Geometry: final body of the model. Coordinates: model frame, mm. Face numbers are marked on the shaded views. A direction names the side the tool comes from. Give positions to 0.01 mm unless a question says otherwise; leave off trailing zeros. Write each loop counter-clockwise with the first axis right and the second up, starting at its lowest first coordinate (ties: lowest second). Pieces come first, ordered by that corner, then holes. Notation, with made-up numbers: M 38,24 L 84,24 A19 ccw 84,54 Z; hole C 81,33 d2. An arc over 180 degrees is marked long. Use one line per item in the form item = value. Start each with the question number.
Item 1: Access query for the marked faces 5, 6 and 7. Directions: +Z, -Z, +X, -X, +Y, -Y. A direction counts if a zero-diameter tool reaches every point of the face in a straight line with its end or side. Return the directions, or none.
Item 2: Material intervals for line 1 along Z through (x, y) = (110, 6.5); line 2 along X through (y, z) = (11.5, -5); line 3 along X through (y, z) = (50.5, -9), sorted ascending. Write a range as from..to.
Item 3: Section query A-A on y = 34.5. Return loops of the section in (x, z), then the cut area to 3 significant figures.
Item 4: Section query C-C on x = -100. Return loops of the section in (y, z).
Item 5: Section query B-B on y = 55. Return loops of the section in (x, z), then the cut area to 3 significant figures.
Item 6: Contact query for flat-ended pins moving along their axis: P1, Ø8, axis at x = 102.5, y = 25.5, coming from the +Z side; P2, Ø1.5, axis at x = 8, y = 66.5, coming from the +Z side; P3, Ø11, axis at y = 8, z = 35.5, coming from the +X side; P4, Ø3, axis at x = -54, z = -25, coming from the +Y side. Output: stop coordinate, or through.
Item 7: Section query D-D on z = 22.5. Return loops of the section in (x, y).
Item 8: Pull-direction query (X, two-part tool) for the marked faces 1, 2, 3 and 4; classes: released by +X, released by -X, zero draft, split by the parting line, or undercut.
from build123d import *

# Parameters (mm, degrees)
SKETCH1_W               = 80
SKETCH1_H               = 80
BOSS_EXTRUDE1_DEPTH     = 80
CUT_EXTRUDE1_DEPTH      = 98.979589711
CUT_EXTRUDE1_DEPTH_BACK = 70
SKETCH2_W               = 60
SKETCH2_H               = 60
SKETCH3_R               = 15
SKETCH3_R_2             = 10
BOSS_EXTRUDE2_DEPTH     = 5
BOSS_EXTRUDE3_DEPTH     = 30
SKETCH5_R               = 15
BOSS_EXTRUDE4_DEPTH     = 10
HOLE1_D                 = 10
HOLE1_CBORE_D           = 20
HOLE1_CBORE_DEPTH       = 15
SKETCH8_W               = 60
SKETCH8_H               = 10
CUT_EXTRUDE2_DEPTH      = 10
SKETCH9_R               = 30
BOSS_EXTRUDE5_DEPTH     = 60
BOSS_EXTRUDE6_DEPTH     = 15
SKETCH11_W              = 30
SKETCH11_H              = 20
CUT_EXTRUDE3_DEPTH      = 180.51323071
SKETCH12_R              = 15
BOSS_EXTRUDE7_DEPTH     = 20
HOLE2_D                 = 20
HOLE3_D                 = 20
HOLE3_DEPTH             = 30
HOLE4_D                 = 20


with BuildPart() as part:
    # Sketch1 → Boss-Extrude1 (new body)
    with BuildSketch(Plane(origin=(0, 0, 0), x_dir=(1, 0, 0), z_dir=(0, 1, 0))):
        Rectangle(SKETCH1_W, SKETCH1_H)
    extrude(amount=BOSS_EXTRUDE1_DEPTH)

    # Sketch2 → Cut-Extrude1 (cut, two sides: drawn at the far end of the back side and taken through both)
    with BuildSketch(Plane.XZ.offset(-CUT_EXTRUDE1_DEPTH_BACK)):
        Rectangle(SKETCH2_W, SKETCH2_H)
    extrude(amount=CUT_EXTRUDE1_DEPTH + CUT_EXTRUDE1_DEPTH_BACK, mode=Mode.SUBTRACT)

    # Sketch3 → Boss-Extrude2 (add)
    with BuildSketch(Plane(origin=(0, 80, 0), x_dir=(1, 0, 0), z_dir=(0, 1, 0))):
        with Locations(Location((0, 0, 0), (0, 0, 270))):
            Circle(SKETCH3_R)
        with Locations(Location((0, 0, 0), (0, 0, 270))):
            Circle(SKETCH3_R_2, mode=Mode.SUBTRACT)
    extrude(amount=BOSS_EXTRUDE2_DEPTH)

    # Sketch4 → Boss-Extrude3 (add)
    with BuildSketch(Plane(origin=(0, 0, 0), x_dir=(1, 0, 0), z_dir=(0, 1, 0))):
        with BuildLine():
            Line((40, 30), (90, 30))
            ThreePointArc((90, 30), (110, 50), (130, 30))
            Line((130, 30), (130, -30))
            ThreePointArc((130, -30), (110, -50), (90, -30))
            Line((90, -30), (40, -30))
            Line((40, -30), (40, 30))
        make_face()
    extrude(amount=BOSS_EXTRUDE3_DEPTH)

    # Sketch5 → Boss-Extrude4 (add)
    with BuildSketch(Plane(origin=(0, 30, 0), x_dir=(1, 0, 0), z_dir=(0, 1, 0))):
        with Locations(Location((110, 30, 0), (0, 0, 270))):
            Circle(SKETCH5_R)
        with Locations(Location((110, -30, 0), (0, 0, 270))):
            Circle(SKETCH5_R)
    extrude(amount=BOSS_EXTRUDE4_DEPTH)

    # Hole1 (through all)
    with Locations(Plane(origin=(0, 40, 0), x_dir=(1, 0, 0), z_dir=(0, 1, 0))):
        with Locations((110, 30), (110, -30)):
            CounterBoreHole(HOLE1_D / 2, HOLE1_CBORE_D / 2, HOLE1_CBORE_DEPTH)

    # Sketch8 → Cut-Extrude2 (cut)
    with BuildSketch(Plane(origin=(0, 30, 0), x_dir=(1, 0, 0), z_dir=(0, 1, 0))):
        with Locations((100, 0)):
            Rectangle(SKETCH8_W, SKETCH8_H)
    extrude(amount=-CUT_EXTRUDE2_DEPTH, mode=Mode.SUBTRACT)



with BuildPart() as body_2:
    # Sketch9 → Boss-Extrude5 (new body)
    with BuildSketch(Plane(origin=(0, 0, 0), x_dir=(1, 0, 0), z_dir=(0, 1, 0))):
        with Locations(Location((-100, 0, 0), (0, 0, 270))):
            Circle(SKETCH9_R)
    extrude(amount=BOSS_EXTRUDE5_DEPTH)


with BuildPart() as part_1:
    add(part.part)

    add(body_2.part)  # Boss-Extrude6 merges body 2
    # Sketch10 → Boss-Extrude6 (add)
    with BuildSketch(Plane(origin=(0, 0, 0), x_dir=(1, 0, 0), z_dir=(0, 1, 0))):
        with BuildLine():
            Line((-40, 40), (-40, -40))
            Line((-40, -40), (-104.747935056, -29.621902584))
            ThreePointArc((-104.747935056, -29.621902584), (-70, 0), (-104.747935056, 29.621902584))
            Line((-104.747935056, 29.621902584), (-40, 40))
        make_face()
    extrude(amount=BOSS_EXTRUDE6_DEPTH)

    # Sketch11 → Cut-Extrude3 (cut, through all)
    with BuildSketch(Plane(origin=(0, 0, -40), x_dir=(-1, 0, 0), z_dir=(0, 0, -1))):
        with Locations((0, 10)):
            Rectangle(SKETCH11_W, SKETCH11_H)
    extrude(amount=-CUT_EXTRUDE3_DEPTH, mode=Mode.SUBTRACT)

    # Sketch12 → Boss-Extrude7 (add)
    with BuildSketch(Plane(origin=(0, 0, -40), x_dir=(-1, 0, 0), z_dir=(0, 0, -1))):
        with Locations(Location((0, 55, 0), (0, 0, 180))):
            Circle(SKETCH12_R)
    extrude(amount=BOSS_EXTRUDE7_DEPTH)

    # Hole2 (through all)
    with Locations(Plane(origin=(0, 80, 0), x_dir=(1, 0, 0), z_dir=(0, 1, 0))):
        with Locations((0, 0)):
            Hole(HOLE2_D / 2)

    # Hole3
    with Locations(Plane(origin=(0, 0, -60), x_dir=(-1, 0, 0), z_dir=(0, 0, -1))):
        with Locations((0, 55)):
            Hole(HOLE3_D / 2, depth=HOLE3_DEPTH)

    # Hole4 (through all)
    with Locations(Plane(origin=(0, 60, 0), x_dir=(1, 0, 0), z_dir=(0, 1, 0))):
        with Locations((-100, 0)):
            Hole(HOLE4_D / 2)


solid = part_1.part
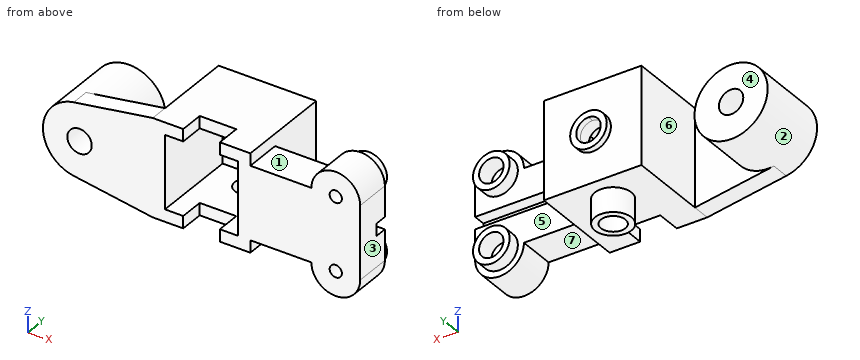
Answer sheet:
q1.face_5 = +Y
q1.face_6 = +Z, -Z, +Y
q1.face_7 = -Z, +Y, -Y
q2.line_1 = -50..-35, -25..25, 35..50
q2.line_2 = -129.58..-108.66, -91.34..-30, 30..130
q2.line_3 = -128.62..-104.36, -95.64..-71.38, -40..-30, 30..40
q3.outline = C -100,0 d60; M -40,-40 L 40,-40 L 40,40 L -40,40 Z; C 110,-30 d30; C 110,30 d30; hole C -100,0 d20; hole M -30,-30 L 30,-30 L 30,30 L -30,30 Z; hole C 110,-30 d20; hole C 110,30 d20
q3.area = 6,100 mm2
q4.outline = M 0,-30.38 L 15,-30.38 L 15,-30 L 60,-30 L 60,-10 L 0,-10 Z; M 0,10 L 60,10 L 60,30 L 15,30 L 15,30.38 L 0,30.38 Z
q5.outline = C -100,0 d60; M -40,-40 L -15,-40 L -15,-60 L -10,-60 L -10,-30 L -30,-30 L -30,30 L 30,30 L 30,-30 L 10,-30 L 10,-60 L 15,-60 L 15,-40 L 40,-40 L 40,40 L -40,40 Z; hole C -100,0 d20
q5.area = 5,310 mm2
q6.P1 = 49.69
q6.P2 = 40
q6.P3 = 130
q6.P4 = 15
q7.outline = M -119.84,0 L -30,0 L -30,70 L 30,70 L 30,0 L 130,0 L 130,30 L 122.99,30 L 122.99,40 L 116.61,40 L 116.61,25 L 103.39,25 L 103.39,40 L 97.01,40 L 97.01,30 L 40,30 L 40,80 L -40,80 L -40,15 L -80.16,15 L -80.16,60 L -119.84,60 Z
q8.face_1 = undercut
q8.face_2 = undercut
q8.face_3 = released by +X
q8.face_4 = zero draft
